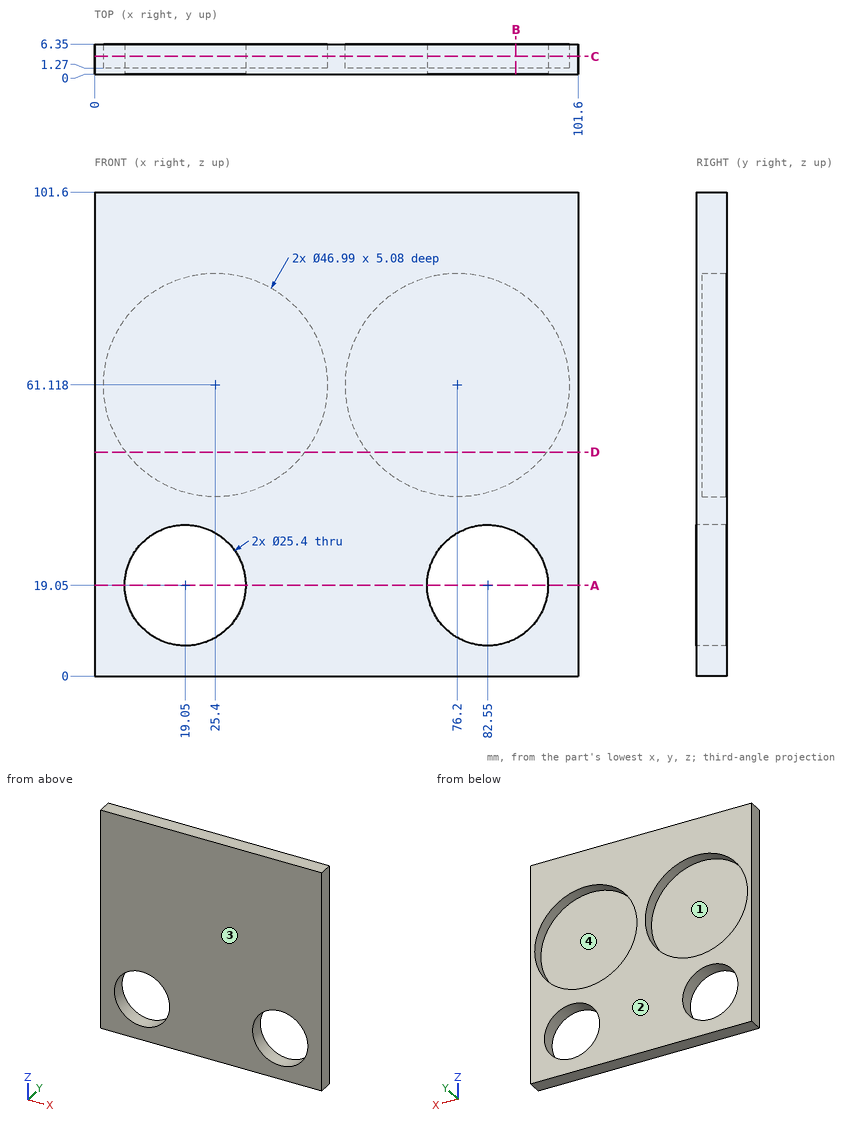
Design review of the part shown in the three views and the two pictorial views. Dimensions are in mm from the part's minimum x, y and z. A direction names the side the tool comes from. Give positions to 0.01 mm unless a question says otherwise; leave off trailing zeros. Loops run counter-clockwise (first coordinate to the right, second up) from the corner with the lowest first, then second, coordinate; pieces in that order, holes last. Notation, with made-up numbers: M -26.5,-21.75 L -3.5,-21.75 A19 cw -3.5,4.25 Z; hole C -31,-30 d10. An arc over 180 degrees is marked long. Answer as a JSON object with one key per item and string values.
Item 1: Mouldability with a two-part tool opening along X and no side actions: class the marked faces 3 and 4 as pulls with the +X half, pulls with the -X half, needs draft (parallel to the pull), parting line crosses it, or undercut.
Output values:
{"face 3": "needs draft", "face 4": "undercut"}
Item 2: We need section D-D (z = 47). State the section outline as (x, y) points.
Output values:
{"outline": "M 0,0 L 101.6,0 L 101.6,6.35 L 94.98,6.35 L 94.98,1.27 L 57.42,1.27 L 57.42,6.35 L 44.18,6.35 L 44.18,1.27 L 6.62,1.27 L 6.62,6.35 L 0,6.35 Z"}
Item 3: We need section A-A (z = 19.05). State the section outline as (x, y) points.
Output values:
{"outline": "M 0,0 L 6.35,0 L 6.35,6.35 L 0,6.35 Z; M 31.75,0 L 69.85,0 L 69.85,6.35 L 31.75,6.35 Z; M 95.25,0 L 101.6,0 L 101.6,6.35 L 95.25,6.35 Z"}
Item 4: We need section C-C (y = 3.75). Count the separate pieces of the cut face and the enclosed holes in it, and give its area (3 significant figures).
Output values:
{"separate pieces": "1", "enclosed holes": "4", "area": "5,840 mm2"}
Item 5: For P1, Ø8, axis at x = 75.5, z = 70.5, coming from the +Y side, flat-tipped, find the tip position at first contact; note if it passes through.
Output values:
{"P1": "stops at y = 1.27"}
Item 6: We need section B-B (x = 88.5). State the section outline as (y, z) points, and give its area (3 significant figures).
Output values:
{"outline": "M 0,0 L 6.35,0 L 6.35,7.83 L 0,7.83 Z; M 0,30.27 L 6.35,30.27 L 6.35,41.1 L 1.27,41.1 L 1.27,81.14 L 6.35,81.14 L 6.35,101.6 L 0,101.6 Z", "area": "299 mm2"}
Item 7: Machinability: for the marked faces 1 and 2, which of the approach directions +Z, -Z, +X, -X, +Y, -Y give a long, thin tool a straight path to every point of the face, cutting with its end or side? Answer none if there is none.
Output values:
{"face 1": "+Y", "face 2": "+Z, -Z, +X, -X, +Y"}
Item 8: Wall thickness on line 1 along X through (y, z) = (3.5, 19.05); line 2 along X through (y, z) = (3, 62); line 3 along Z through (x, y) = (19.05, 3.75): over which ranges is each line inside the solid? List them lowest first.
Output values:
{"line 1": "x = 0 to 6.35, 31.75 to 69.85, 95.25 to 101.6", "line 2": "x = 0 to 1.92, 48.88 to 52.72, 99.68 to 101.6", "line 3": "z = 0 to 6.35, 31.75 to 38.5, 83.74 to 101.6"}
